```python
from build123d import *

# Parameters (mm, degrees)
BOSS_EXTRUDE1_DEPTH      = 5
BOSS_EXTRUDE1_DEPTH_BACK = 5
SKETCH7_R                = 2.788241988
SKETCH7_R_2              = 2.75
BOSS_EXTRUDE2_REACH      = 46.511
CUT_EXTRUDE3_REACH       = 76.833
SKETCH14_W               = 13
SKETCH14_H               = 1.848424097
SKETCH15_R               = 1.45
CUT_EXTRUDE4_DEPTH       = 3
CUT_EXTRUDE5_REACH       = 56.263
SKETCH16_R               = 2
FILLET1_R                = 0.5


with BuildPart() as part:
    # Sketch7 → Boss-Extrude1 (new, two sides: drawn at the far end of the back side and taken through both)
    with BuildSketch(Plane.XY.offset(-BOSS_EXTRUDE1_DEPTH_BACK)):
        with BuildLine():
            Line((30, 8), (30, 0))
            Line((30, 0), (60, 0))
            Line((60, 0), (60, 32.5))
            Line((60, 32.5), (47, 32.5))
            Line((47, 32.5), (47, 25))
            ThreePointArc((47, 25), (42.02081528, 12.97918472), (30, 8))
        make_face()
        with Locations((53, 7)):
            Circle(SKETCH7_R, mode=Mode.SUBTRACT)
        with Locations((53, 25)):
            Circle(SKETCH7_R_2, mode=Mode.SUBTRACT)
    extrude(amount=BOSS_EXTRUDE1_DEPTH + BOSS_EXTRUDE1_DEPTH_BACK)

    # Boss-Extrude2: up to this face of the body (flat: up to its plane)
    boss_extrude2_end = Plane(part.part.faces().sort_by_distance((47, 28.75, 0))[0])
    # Sketch8 → Boss-Extrude2 (add, up to the picked face)
    with BuildSketch(Plane(origin=(60, 0, 0), x_dir=(0, 0, -1), z_dir=(1, 0, 0)), mode=Mode.PRIVATE) as boss_extrude2_sk1:
        with BuildLine():
            Line((7.770224858, 6.297913321), (7.77021842, 8.534450023))
            ThreePointArc((7.77021842, 8.534450023), (7.172653823, 9.41960576), (6.160789156, 9.761240102))
            Line((6.160789156, 9.761240102), (6.049331791, 9.761231883))
            ThreePointArc((6.049331791, 9.761231883), (5.467920254, 9.629507338), (5, 9.260127632))
            Line((5, 9.260127632), (5, 16.139290416))
            ThreePointArc((5, 16.139290416), (5.467793594, 15.770087219), (6.049012407, 15.638456908))
            Line((6.049012407, 15.638456908), (6.160787586, 15.638456908))
            ThreePointArc((6.160787586, 15.638456908), (7.114683416, 16.033573497), (7.509800005, 16.987469327))
            Line((7.509800005, 16.987469327), (7.509800005, 19.102089972))
            ThreePointArc((7.509800005, 19.102089972), (7.80571774, 19.4939479), (8.26359849, 19.316563682))
            Line((8.26359849, 19.316563682), (11.653749185, 15.934160795))
            ThreePointArc((11.653749185, 15.934160795), (12.207484328, 15.158579301), (12.477275173, 14.244597811))
            Line((12.477275173, 14.244597811), (12.625702616, 11.128406988))
            ThreePointArc((12.625702616, 11.128406988), (12.368540167, 10.154062981), (11.790945096, 9.328313198))
            Line((11.790945096, 9.328313198), (8.480768071, 6.02568809))
            ThreePointArc((8.480768071, 6.02568809), (8.03188202, 5.917454844), (7.770224858, 6.297913321))
        make_face()
    boss_extrude2_tool1 = split(extrude(boss_extrude2_sk1.sketch, amount=-BOSS_EXTRUDE2_REACH, mode=Mode.PRIVATE), bisect_by=boss_extrude2_end, keep=Keep.BOTH, mode=Mode.PRIVATE)
    # Sketch8 → Boss-Extrude2 (add, up to the picked face)
    with BuildSketch(Plane(origin=(60, 0, 0), x_dir=(0, 0, -1), z_dir=(1, 0, 0)), mode=Mode.PRIVATE) as boss_extrude2_sk2:
        with BuildLine():
            Line((30.631565341, 16.79432062), (30.631565341, 23.861822271))
            ThreePointArc((30.631565341, 23.861822271), (29.994638774, 24.994670327), (28.861778916, 25.631575903))
            Line((28.861778916, 25.631575903), (21.563333135, 25.631575903))
            ThreePointArc((21.563333135, 25.631575903), (20.893881396, 25.140801297), (20.6385, 24.350987593))
            Line((20.6385, 24.350987593), (20.6385, 24.239212407))
            ThreePointArc((20.6385, 24.239212407), (21.033616586, 23.285316586), (21.987512407, 22.8902))
            Line((21.987512407, 22.8902), (24.176788598, 22.8902))
            ThreePointArc((24.176788598, 22.8902), (24.854992901, 22.436757749), (24.695146796, 21.63674514))
            Line((24.695146796, 21.63674514), (21.386383353, 18.335543623))
            ThreePointArc((21.386383353, 18.335543623), (20.461951665, 17.745653619), (19.375383804, 17.597618335))
            Line((19.375383804, 17.597618335), (16.024616196, 17.597618335))
            ThreePointArc((16.024616196, 17.597618335), (14.938048335, 17.745653619), (14.013616647, 18.335543623))
            Line((14.013616647, 18.335543623), (10.704853204, 21.63674514))
            ThreePointArc((10.704853204, 21.63674514), (10.545007099, 22.436757749), (11.223211402, 22.8902))
            Line((11.223211402, 22.8902), (13.412487593, 22.8902))
            ThreePointArc((13.412487593, 22.8902), (14.366383414, 23.285316586), (14.7615, 24.239212407))
            Line((14.7615, 24.239212407), (14.7615, 24.350987593))
            ThreePointArc((14.7615, 24.350987593), (14.506118604, 25.140801297), (13.836666865, 25.631575903))
            Line((13.836666865, 25.631575903), (6.538221084, 25.631575903))
            ThreePointArc((6.538221084, 25.631575903), (5.64574769, 25.205085259), (5, 24.455810309))
            Line((5, 24.455810309), (5, 30.651575903))
            Line((5, 30.651575903), (35.719846982, 30.651575903))
            Line((35.719846982, 30.651575903), (35.719846982, 25.680977676))
            Line((35.719846982, 25.680977676), (35.719846982, 8.441932485))
            Line((35.719846982, 8.441932485), (30.699526538, 8.441932485))
            Line((30.699526538, 8.441932485), (30.4, 9.260127632))
            ThreePointArc((30.4, 9.260127632), (29.932079746, 9.629507338), (29.350668209, 9.761231883))
            Line((29.350668209, 9.761231883), (29.239210844, 9.761240102))
            ThreePointArc((29.239210844, 9.761240102), (28.227346177, 9.41960576), (27.62978158, 8.534450023))
            Line((27.62978158, 8.534450023), (27.629775142, 6.29790377))
            ThreePointArc((27.629775142, 6.29790377), (27.368113521, 5.917453135), (26.919231929, 6.02568809))
            Line((26.919231929, 6.02568809), (23.609054904, 9.328313198))
            ThreePointArc((23.609054904, 9.328313198), (23.031459833, 10.154062981), (22.774297384, 11.128406988))
            Line((22.774297384, 11.128406988), (22.922724827, 14.244597811))
            ThreePointArc((22.922724827, 14.244597811), (23.192519205, 15.158586549), (23.746262232, 15.934172186))
            Line((23.746262232, 15.934172186), (27.13640151, 19.316563682))
            ThreePointArc((27.13640151, 19.316563682), (27.594282383, 19.493947864), (27.890199995, 19.102089715))
            Line((27.890199995, 19.102089715), (27.890199995, 16.987469327))
            ThreePointArc((27.890199995, 16.987469327), (28.285316584, 16.033573497), (29.239212414, 15.638456908))
            Line((29.239212414, 15.638456908), (29.350987593, 15.638456908))
            ThreePointArc((29.350987593, 15.638456908), (29.932206406, 15.770087219), (30.4, 16.139290416))
            Line((30.4, 16.139290416), (30.631565341, 16.79432062))
        make_face()
    boss_extrude2_tool2 = split(extrude(boss_extrude2_sk2.sketch, amount=-BOSS_EXTRUDE2_REACH, mode=Mode.PRIVATE), bisect_by=boss_extrude2_end, keep=Keep.BOTH, mode=Mode.PRIVATE)
    add(boss_extrude2_tool1.solids().sort_by(Axis((60, 12.678642, -8.819589), (-1, 0, 0)))[0])
    add(boss_extrude2_tool2.solids().sort_by(Axis((60, 21.642021, -23.841508), (-1, 0, 0)))[0])

    # Sketch14 → Cut-Extrude3 (cut, up to next)
    with BuildSketch(Plane(origin=(0, 0, -5), x_dir=(-1, 0, 0), z_dir=(0, 0, -1)), mode=Mode.PRIVATE) as cut_extrude3_sk1:
        with Locations((-53.5, 31.575787952)):
            Rectangle(SKETCH14_W, SKETCH14_H)
    cut_extrude3_tool1 = extrude(cut_extrude3_sk1.sketch, amount=-CUT_EXTRUDE3_REACH, mode=Mode.PRIVATE) & part.part
    add(cut_extrude3_tool1.solids().sort_by_distance((53.5, 31.575788, -5))[0], mode=Mode.SUBTRACT)

    # Sketch15 → Cut-Extrude4 (cut)
    with BuildSketch(Plane.ZY.offset(-30)):
        with Locations(Location((0, 4, 0), (0, 0, 270))):
            Circle(SKETCH15_R)
    extrude(amount=-CUT_EXTRUDE4_DEPTH, mode=Mode.SUBTRACT)

    # Sketch16 → Cut-Extrude5 (cut, up to next)
    with BuildSketch(Plane.ZY.offset(-33), mode=Mode.PRIVATE) as cut_extrude5_sk1:
        with Locations(Location((0, 4, 0), (0, 0, 270))):
            Circle(SKETCH16_R)
    cut_extrude5_tool1 = extrude(cut_extrude5_sk1.sketch, amount=-CUT_EXTRUDE5_REACH, mode=Mode.PRIVATE) & part.part
    add(cut_extrude5_tool1.solids().sort_by_distance((33, 4, 0))[0], mode=Mode.SUBTRACT)

    # Fillet1
    fillet1_edges = [part.edges().sort_by_distance(p)[0] for p in [
        (33, 6, 0),
    ]]
    fillet(fillet1_edges, radius=FILLET1_R)


solid = part.part
```
Input: part model. Units: mm. Frame: model coordinates. A direction names the side the tool comes from. Coordinates: 2 decimals unless noted, no trailing zeros. Loops run counter-clockwise (first coordinate to the right, second up) from the corner with the lowest first, then second, coordinate; pieces in that order, holes last.
Q1. Section D-D, the plane x = 53. Give the number of separate pieces and of enclosed holes in the cut face, and give its area (3 significant figures).
Results are:
separate pieces: 3
enclosed holes: 0
area: 638 mm2
Q2. Line query: line 1 along Y through (x, z) = (53, -2.25); line 2 along Z through (x, y) = (54.5, 4); line 3 along Y through (x, z) = (53, 0). Output: solid intervals per line, ascending.
Results are:
line 1: y = 0 to 4.21, 9.79 to 22.25, 27.75 to 30.65
line 2: z = -5 to -2, 2 to 5
line 3: y = 0 to 2, 9.79 to 22.25, 27.75 to 30.65
Q3. Mould query, pull axis Y, two halves, no side actions, for faces 5 (the flat face through (47, 21, -20)), 6 (the cylindrical face through (53.591, 22.426, -10.54)), 7 (the cylindrical face through (53.591, 17.751, -20.476)). Classes: +Y half, -Y half, draft (parallel to the pull), parting line (faces both ways), or undercut.
Results are:
face 5: draft
face 6: undercut
face 7: -Y half
Q4. Section C-C, the plane y = 7.5. Return the cut outline in (x, z), and give its area (3 significant figures).
Results are:
outline: (30, -5) - (50.26, -5) - (50.26, 5) - (30, 5) - close; (47, -27.63) - (60, -27.63) - (60, -25.44) - (47, -25.44) - close; (47, -9.96) - (60, -9.96) - (60, -7.77) - (47, -7.77) - close; (55.74, -5) - (60, -5) - (60, 5) - (55.74, 5) - close
area: 302 mm2
Q5. Section A-A, the plane z = -4.5. Return the cut outline in (x, y).
Results are:
outline: (30, 0) - (60, 0) - (60, 30.65) - (47, 30.65) - (47, 25) arc R17 cw to (30, 8) - close; hole circle Ø5.58 at (53, 7); hole circle Ø5.5 at (53, 25)
Q6. Set-up query: faces 1 (the flat face through (54, 20, -35.72)), 2 (the cylindrical face through (52.637, 9.765, -0.07)), 3 (the cylindrical face through (53.591, 15.774, -5.46)), 4 (the flat face through (54, 17.598, -18)). Return all of +Z, -Z, +X, -X, +Y, -Y with unobstructed straight access to the full face (end or side cutting, diameter ignored); none if empty.
Results are:
face 1: -Z, +X, -X, +Y, -Y
face 2: +Z
face 3: +X, -X
face 4: +X, -X, -Y
Q7. Section B-B, the plane z = 0. Return the cut outline in (x, y).
Results are:
outline: (30, 0) - (60, 0) - (60, 2) - (33.5, 2) arc R0.5 cw to (33, 2.5) - (33, 2.55) - (30, 2.55) - close; (30, 5.45) - (33, 5.45) - (33, 5.5) arc R0.5 cw to (33.5, 6) - (50.4, 6) arc R2.79 cw (long way) to (55.6, 6) - (60, 6) - (60, 30.65) - (47, 30.65) - (47, 25) arc R17 cw to (30, 8) - close; hole circle Ø5.5 at (53, 25)
Q8. Contact query for flat-ended pins moving along their axis: pin 1 (1.5 mm diameter, centred on x = 38.5, z = -1.5, fed in from +Y); pin 2 (8 mm diameter, centred on y = 19, z = -28.5, fed in from +X); pin 3 (8.5 mm diameter, centred on y = 10, z = -9.5, fed in from -X); pin 4 (7.5 mm diameter, centred on y = 13.5, z = -18.5, fed in from -X). Output: stop coordinate, or through.
Results are:
pin 1: stops at y = 10.74
pin 2: stops at x = 60
pin 3: stops at x = 47
pin 4: passes through
